Build history of the part. All positions in model axes, mm. Face numbers are marked on the shaded views. A direction names the side the tool comes from. Coordinates: 2 decimals unless noted, no trailing zeros. Loops run counter-clockwise (first coordinate to the right, second up) from the corner with the lowest first, then second, coordinate; pieces in that order, holes last.
(1) Slice it at B-B (x = -15.5). Give the cut face in (y, z), and give its area (3 significant figures).
(2) Slice it at C-C (z = -17). Give the cut face in (x, y), and give its area (3 significant figures).
(3) Wall check: L1, parallel to Y at x = 4.5, z = -9; L2, parallel to Z at x = -8.5, y = -4.75. Give the ranges that are in metal, low to high.
(4) Slice it at D-D (z = 4). Give the cut face in (x, y), and give its area (3 significant figures).
(5) Slice it at A-A (y = -3). Give the cut face in (x, z), and give its area (3 significant figures).
(6) Flat gauge pins, fed straight in: P1, Ø10, axis at y = -13.5, z = -10.5, coming from the -X side; P2, Ø6, axis at x = 21, z = 19.5, coming from the +Y side; P3, Ø2.5, axis at y = -15, z = -15, coming from the +X side; P4, Ø1.5, axis at y = -2, z = 20, coming from the -X side. Where does each tip first touch, or does it go through?
(7) Tool access for the marked faces 5, 6 and 7: list every direction of +Z, -Z, +X, -X, +Y, -Y with a clear straight run to the whole face (end or side of a thin tool).
(8) Two-plate mould, pull along Y, no slides. Class the marked faces 1, 2, 3 and 4: pulls with the +Y half, pulls with the -Y half, needs draft (parallel to the pull), parting line crosses it, or undercut.
from build123d import *

# Parameters (mm, degrees)
SKETCH_1_W           = 19
SKETCH_1_H           = 19
SKETCH_1_W_2         = 55
SKETCH_1_H_2         = 7
EXTRUDE_1_DEPTH      = 21
SKETCH_1_3_W         = 13
SKETCH_1_3_H         = 13
CUT_EXTRUDE_1_DEPTH  = 21
SKETCH_1_12_W        = 19
SKETCH_1_12_H        = 19
SKETCH_1_12_W_2      = 14.6
SKETCH_1_12_H_2      = 14.6
CUT_EXTRUDE_6_DEPTH  = 18
CUT_EXTRUDE_7_DEPTH  = 14.5
SKETCH_4_W           = 3.5
SKETCH_4_H           = 7
SKETCH_4_W_2         = 3.504900739
EXTRUDE_2_DEPTH      = 27.5
SKETCH_10_W          = 1
SKETCH_10_H          = 7
EXTRUDE_4_DEPTH      = 55
SKETCH_14_W          = 1
SKETCH_14_H          = 7
EXTRUDE_6_DEPTH      = 55
CUT_EXTRUDE_17_DEPTH = 2.3
CUT_EXTRUDE_18_DEPTH = 2.3
CUT_EXTRUDE_19_DEPTH = 2.3
CUT_EXTRUDE_20_DEPTH = 2.3


with BuildPart() as part:
    # Sketch 1 → Extrude 1 (new body, symmetric)
    with BuildSketch(Plane.XY):
        Rectangle(SKETCH_1_W, SKETCH_1_H)
        with Locations((0, -13)):
            Rectangle(SKETCH_1_W_2, SKETCH_1_H_2)
    extrude(amount=EXTRUDE_1_DEPTH, both=True)

    # Sketch 1_3 → Cut-Extrude 1 (cut, symmetric)
    with BuildSketch(Plane.XY):
        Rectangle(SKETCH_1_3_W, SKETCH_1_3_H)
    extrude(amount=CUT_EXTRUDE_1_DEPTH, both=True, mode=Mode.SUBTRACT)

    # Sketch 1_12 → Cut-Extrude 6 (cut, symmetric)
    with BuildSketch(Plane.XY):
        Rectangle(SKETCH_1_12_W, SKETCH_1_12_H)
        Rectangle(SKETCH_1_12_W_2, SKETCH_1_12_H_2, mode=Mode.SUBTRACT)
    extrude(amount=CUT_EXTRUDE_6_DEPTH, both=True, mode=Mode.SUBTRACT)

    # Sketch 1_13 → Cut-Extrude 7 (cut, symmetric)
    with BuildSketch(Plane.XY):
        Polygon((9.5, -9.5), (-9.5, -9.5), (-27.5, -9.5), (-27.5, -16.5), (27.5, -16.5), (27.5, -9.5), align=None)
    extrude(amount=CUT_EXTRUDE_7_DEPTH, both=True, mode=Mode.SUBTRACT)

    # Sketch 4 → Extrude 2 (add, symmetric)
    with BuildSketch(Plane(origin=(0, 0, 0), x_dir=(0, 0, -1), z_dir=(1, 0, 0))):
        with Locations((22.75, -13)):
            Rectangle(SKETCH_4_W, SKETCH_4_H)
        with Locations((-22.752450369, -13)):
            Rectangle(SKETCH_4_W_2, SKETCH_4_H)
    extrude(amount=EXTRUDE_2_DEPTH, both=True)

    # Sketch 10 → Extrude 4 (add)
    with BuildSketch(Plane(origin=(27.5, 0, 0), x_dir=(0, 0, -1), z_dir=(1, 0, 0))):
        with Locations((-25.004900739, -13)):
            Rectangle(SKETCH_10_W, SKETCH_10_H)
        with Locations((-14, -13)):
            Rectangle(SKETCH_10_W, SKETCH_10_H)
    extrude(amount=-EXTRUDE_4_DEPTH)

    # Sketch 14 → Extrude 6 (add)
    with BuildSketch(Plane(origin=(27.5, 0, 0), x_dir=(0, 0, -1), z_dir=(1, 0, 0))):
        with Locations((14, -13)):
            Rectangle(SKETCH_14_W, SKETCH_14_H)
        with Locations((25, -13)):
            Rectangle(SKETCH_14_W, SKETCH_14_H)
    extrude(amount=-EXTRUDE_6_DEPTH)

    # Sketch 15 → Cut-Extrude 17 (cut)
    with BuildSketch(Plane(origin=(0, 0, -25.5), x_dir=(-1, 0, 0), z_dir=(0, 0, -1))):
        Polygon((-27.5, -9.5), (-27.5, -16.5), (-24.36, -16.5), (-24.36, -12.5), (-22.86, -12.5), (-21.36, -12.5), (-21.36, -16.5), (-19.28, -16.5), (-19.28, -12.5), (-17.78, -12.5), (-16.28, -12.5), (-16.28, -16.5), (-14.2, -16.5), (-14.2, -12.5), (-12.7, -12.5), (-11.2, -12.5), (-11.2, -16.5), (-9.12, -16.5), (-9.12, -12.5), (-7.62, -12.5), (-6.12, -12.5), (-6.12, -16.5), (-4.04, -16.5), (-4.04, -12.5), (-2.54, -12.5), (-1.04, -12.5), (-1.04, -16.5), (1.04, -16.5), (1.04, -12.5), (2.54, -12.5), (4.04, -12.5), (4.04, -16.5), (6.12, -16.5), (6.12, -12.5), (7.62, -12.5), (9.12, -12.5), (9.12, -16.5), (11.2, -16.5), (11.2, -12.5), (12.7, -12.5), (14.2, -12.5), (14.2, -16.5), (16.28, -16.5), (16.28, -12.5), (17.78, -12.5), (19.28, -12.5), (19.28, -16.5), (21.36, -16.5), (21.36, -12.5), (22.86, -12.5), (24.36, -12.5), (24.36, -16.5), (27.5, -16.5), (27.5, -9.5), align=None)
    extrude(amount=-CUT_EXTRUDE_17_DEPTH, mode=Mode.SUBTRACT)

    # Sketch 16 → Cut-Extrude 18 (cut)
    with BuildSketch(Plane(origin=(0, 0, 13.5), x_dir=(-1, 0, 0), z_dir=(0, 0, -1))):
        Polygon((27.5, -9.5), (-27.5, -9.5), (-27.5, -16.5), (-24.36, -16.5), (-24.36, -12.5), (-21.36, -12.5), (-21.36, -16.5), (-19.28, -16.5), (-19.28, -12.5), (-16.28, -12.5), (-16.28, -16.5), (-14.2, -16.5), (-14.2, -12.5), (-11.2, -12.5), (-11.2, -16.5), (-9.12, -16.5), (-9.12, -12.5), (-6.12, -12.5), (-6.12, -16.5), (-4.04, -16.5), (-4.04, -12.5), (-1.04, -12.5), (-1.04, -16.5), (1.04, -16.5), (1.04, -12.5), (4.04, -12.5), (4.04, -16.5), (6.12, -16.5), (6.12, -12.5), (9.12, -12.5), (9.12, -16.5), (11.2, -16.5), (11.2, -12.5), (14.2, -12.5), (14.2, -16.5), (16.28, -16.5), (16.28, -12.5), (19.28, -12.5), (19.28, -16.5), (21.36, -16.5), (21.36, -12.5), (24.36, -12.5), (24.36, -16.5), (27.5, -16.5), align=None)
    extrude(amount=-CUT_EXTRUDE_18_DEPTH, mode=Mode.SUBTRACT)

    # Sketch 17 → Cut-Extrude 19 (cut)
    with BuildSketch(Plane.XY.offset(-13.5)):
        Polygon((24.36, -16.5), (27.5, -16.5), (27.5, -9.5), (-27.5, -9.5), (-27.5, -16.5), (-24.36, -16.5), (-24.36, -12.5), (-21.36, -12.5), (-21.36, -16.5), (-19.28, -16.5), (-19.28, -12.5), (-16.28, -12.5), (-16.28, -16.5), (-14.2, -16.5), (-14.2, -12.5), (-11.2, -12.5), (-11.2, -16.5), (-9.12, -16.5), (-9.12, -12.5), (-6.12, -12.5), (-6.12, -16.5), (-4.04, -16.5), (-4.04, -12.5), (-1.04, -12.5), (-1.04, -16.5), (1.04, -16.5), (1.04, -12.5), (4.04, -12.5), (4.04, -16.5), (6.12, -16.5), (6.12, -12.5), (9.12, -12.5), (9.12, -16.5), (11.2, -16.5), (11.2, -12.5), (14.2, -12.5), (14.2, -16.5), (16.28, -16.5), (16.28, -12.5), (19.28, -12.5), (19.28, -16.5), (21.36, -16.5), (21.36, -12.5), (24.36, -12.5), align=None)
    extrude(amount=-CUT_EXTRUDE_19_DEPTH, mode=Mode.SUBTRACT)

    # Sketch 18 → Cut-Extrude 20 (cut)
    with BuildSketch(Plane.XY.offset(25.504900739)):
        Polygon((24.36, -16.5), (27.5, -16.5), (27.5, -9.5), (-27.5, -9.5), (-27.5, -16.5), (-24.36, -16.5), (-24.36, -12.5), (-21.36, -12.5), (-21.36, -16.5), (-19.28, -16.5), (-19.28, -12.5), (-16.28, -12.5), (-16.28, -16.5), (-14.2, -16.5), (-14.2, -12.5), (-11.2, -12.5), (-11.2, -16.5), (-9.12, -16.5), (-9.12, -12.5), (-6.12, -12.5), (-6.12, -16.5), (-4.04, -16.5), (-4.04, -12.5), (-1.04, -12.5), (-1.04, -16.5), (1.04, -16.5), (1.04, -12.5), (4.04, -12.5), (4.04, -16.5), (6.12, -16.5), (6.12, -12.5), (9.12, -12.5), (9.12, -16.5), (11.2, -16.5), (11.2, -12.5), (14.2, -12.5), (14.2, -16.5), (16.28, -16.5), (16.28, -12.5), (19.28, -12.5), (19.28, -16.5), (21.36, -16.5), (21.36, -12.5), (24.36, -12.5), align=None)
    extrude(amount=-CUT_EXTRUDE_20_DEPTH, mode=Mode.SUBTRACT)


solid = part.part
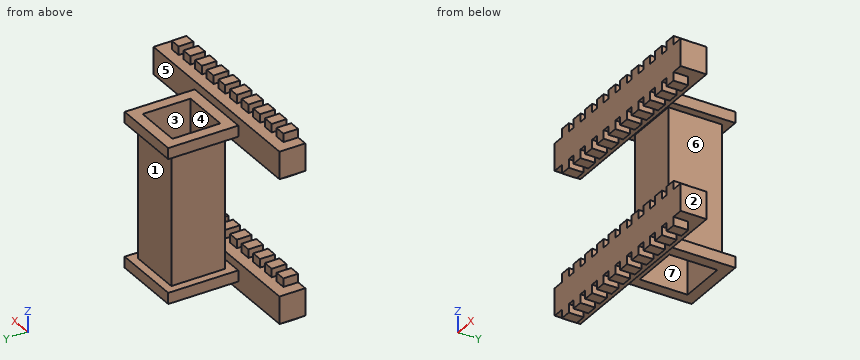
Response values:
1. outline: (-16.5, -23.2) - (-9.5, -23.2) - (-9.5, -15.8) - (-16.5, -15.8) - close; (-16.5, 15.8) - (-9.5, 15.8) - (-9.5, 23.2) - (-16.5, 23.2) - close
1. area: 104 mm2
2. outline: (-27.5, -16.5) - (27.5, -16.5) - (27.5, -9.5) - (-27.5, -9.5) - close; (-7.3, -7.3) - (7.3, -7.3) - (7.3, 7.3) - (-7.3, 7.3) - close; hole (-6.5, -6.5) - (6.5, -6.5) - (6.5, 6.5) - (-6.5, 6.5) - close
2. area: 429 mm2
3. L1: y = -7.3 to -6.5, 6.5 to 7.3
3. L2: z = -21 to -18, 18 to 21
4. outline: (-7.3, -7.3) - (7.3, -7.3) - (7.3, 7.3) - (-7.3, 7.3) - close; hole (-6.5, -6.5) - (6.5, -6.5) - (6.5, 6.5) - (-6.5, 6.5) - close
4. area: 44.2 mm2
5. outline: (-9.5, -21) - (-6.5, -21) - (-6.5, 21) - (-9.5, 21) - (-9.5, 18) - (-7.3, 18) - (-7.3, -18) - (-9.5, -18) - close; (6.5, -21) - (9.5, -21) - (9.5, -18) - (7.3, -18) - (7.3, 18) - (9.5, 18) - (9.5, 21) - (6.5, 21) - close
5. area: 93.6 mm2
6. P1: stops at x = -24.36
6. P2: stops at y = -9.5
6. P3: stops at x = 27.5
6. P4: stops at x = -9.5
7. face 5: none
7. face 6: +X, +Y
7. face 7: +Z, -Z
8. face 1: pulls with the +Y half
8. face 2: needs draft
8. face 3: undercut
8. face 4: undercut
